Work out the finished part from the listing and answer in its coordinate system (mm). Coordinates: 2 decimals unless noted, no trailing zeros. Write each loop counter-clockwise with the first axis right and the second up, starting at its lowest first coordinate (ties: lowest second). Pieces come first, ordered by that corner, then holes. Notation, with made-up numbers: (38, -29.75) - (63, -29.75) arc R29 ccw to (63, -8.75) - close; hole circle Ø2 at (-26, 30). An arc over 180 degrees is marked (long way). Use one line per item in the form item = value. Start each with the question number.
Item 1: A cutting plane is placed at C-C (x = 8.5). Write down the section's boundary in (y, z).
Item 2: A cutting plane is placed at B-B (z = 0.8). Write down the section's boundary in (x, y), then the cut area to 3 significant figures.
Item 3: Consider probe 1 along X at (y, z) = (29, 1.5); probe 2 along X at (y, z) = (-4.5, 2.1); probe 3 along Y at (x, z) = (9.25, 1.95). Determine where each line is inside the solid, lowest interval first.
Item 4: Given pin 1 (1.5 mm diameter, centred on y = 9, z = 2, fed in from -X); pin 2 (0.9 mm diameter, centred on y = 27.5, z = 1.5, fed in from +X); pin 3 (4 mm diameter, centred on x = -0.5, y = 4.5, fed in from -Z); pin 4 (0.8 mm diameter, centred on x = 5, z = 1, fed in from +Y), each flat-ended and moving along its own axis, determine where each tip first touches the part or whether it passes through.
Item 5: A cutting plane is placed at D-D (y = -32.5). Write down the section's boundary in (x, z), then the cut area to 3 significant figures.
Item 6: A cutting plane is placed at A-A (y = 34). Write down the section's boundary in (x, z), then the cut area to 3 significant figures.
from build123d import *

# Parameters (mm, degrees)
EXTRUDE_1_DEPTH     = 3
SKETCH_2_W          = 3
SKETCH_2_H          = 36.495999937
CUT_EXTRUDE_1_DEPTH = 3
SKETCH_3_W          = 3
SKETCH_3_H          = 3
EXTRUDE_2_DEPTH     = 3
SKETCH_4_W          = 8
SKETCH_4_H          = 3.1
EXTRUDE_3_DEPTH     = 3


with BuildPart() as part:
    # 스케치1 → 보스-돌출1 (new body)
    with BuildSketch(Plane.XY):
        Polygon((-4.5, 39.545999937), (4.5, 39.545999937), (4.5, -30.445999937), (7, -30.445999937), (7, -39.545999937), (4, -39.545999937), (4, -33.445999937), (-4, -33.445999937), (-4, -39.545999937), (-7, -39.545999937), (-7, -30.445999937), (-4.5, -30.445999937), align=None)
    extrude(amount=EXTRUDE_1_DEPTH)

    # 스케치2 → 컷-돌출1 (cut)
    with BuildSketch(Plane.XY.offset(3)):
        with Locations((0, 21.297999969)):
            Rectangle(SKETCH_2_W, SKETCH_2_H)
    extrude(amount=-CUT_EXTRUDE_1_DEPTH, mode=Mode.SUBTRACT)

    # 스케치3 → 보스-돌출2 (add)
    with BuildSketch(Plane.XY.offset(3)):
        with Locations((-8.5, -35.045999937)):
            Rectangle(SKETCH_3_W, SKETCH_3_H)
        with Locations((8.5, -35.045999937)):
            Rectangle(SKETCH_3_W, SKETCH_3_H)
    extrude(amount=-EXTRUDE_2_DEPTH)

    # 스케치4 → 보스-돌출3 (add)
    with BuildSketch(Plane.XY.offset(3)):
        with Locations((0, -34.995999937)):
            Rectangle(SKETCH_4_W, SKETCH_4_H)
    extrude(amount=-EXTRUDE_3_DEPTH)


solid = part.part
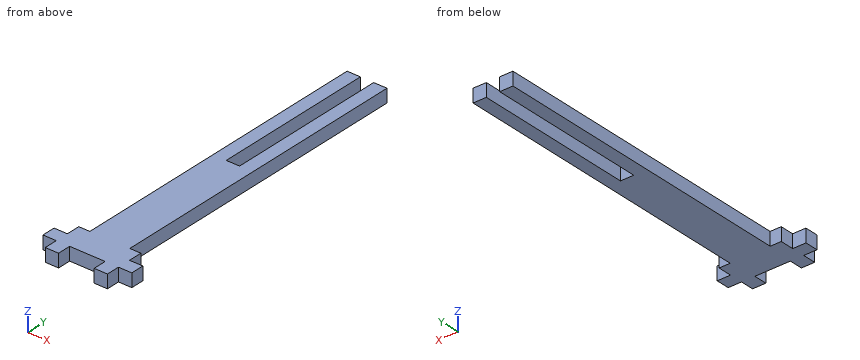
Answer:
q1.outline = (-36.55, 0) - (-33.55, 0) - (-33.55, 3) - (-36.55, 3) - close
q2.outline = (-10, -36.55) - (-7, -36.55) - (-7, -39.55) - (-4, -39.55) - (-4, -36.55) - (4, -36.55) - (4, -39.55) - (7, -39.55) - (7, -36.55) - (10, -36.55) - (10, -33.55) - (7, -33.55) - (7, -30.45) - (4.5, -30.45) - (4.5, 39.55) - (1.5, 39.55) - (1.5, 3.05) - (-1.5, 3.05) - (-1.5, 39.55) - (-4.5, 39.55) - (-4.5, -30.45) - (-7, -30.45) - (-7, -33.55) - (-10, -33.55) - close
q2.area = 642 mm²
q3.probe_1 = -4.5 to -1.5, 1.5 to 4.5
q3.probe_2 = -4.5 to 4.5
q3.probe_3 = -36.55 to -33.55
q4.pin_1 = -4.5
q4.pin_2 = 4.5
q4.pin_3 = 0
q4.pin_4 = -30.45
q5.outline = (-7, 0) - (7, 0) - (7, 3) - (-7, 3) - close
q5.area = 42.0 mm²
q6.outline = (-4.5, 0) - (-1.5, 0) - (-1.5, 3) - (-4.5, 3) - close; (1.5, 0) - (4.5, 0) - (4.5, 3) - (1.5, 3) - close
q6.area = 18.0 mm²
